Can you work these out from the model? Positions are in its coordinate system, mm. Coordinates: 2 decimals unless noted, no trailing zeros. Order: outer loops, then holes, each group sorted by start corner. A loop starts at its lowest first (then second) coordinate and runs counter-clockwise, first axis right, second up. Notation, with made-up numbers: (43.25, 21.5) -> (101.25, 21.5) arc R10 cw to (101.25, 40.5) -> close; hole circle Ø8 at (-14, 80). An arc over 180 degrees is marked (long way). Return JSON: item names as keys, results as strings. Group by question number.
1) If we section it at B-B, the plane x = 4: Please give me the cut outline in (y, z), then the cut area to 3 significant figures.
2) If we section it at D-D, the plane x = -3.7: Please give me the cut outline in (y, z).
3) If we section it at C-C, the plane z = 1.1: Please give me the cut outline in (x, y).
4) If we section it at A-A, the plane y = -8: Please give me the cut outline in (x, z).
5) If I drill on probe 1 along Y at (x, z) = (-3.7, 1.2); probe 2 along Y at (x, z) = (-3.5, 1.65); probe 3 along X at (y, z) = (13, 0.5), over which ranges is the centre line in solid material (lowest first)? Write a range as from..to.
6) For pin 1 (1 mm diameter, centred on x = -5, z = 2, fed in from +Y); pin 2 (4 mm diameter, centred on x = -3.7, y = 4, fed in from +Z); pin 3 (2.5 mm diameter, centred on x = -3, y = -17, fed in from -Z), each with a flat end and sliding along its axis, tell me the tip position at first contact or that it passes through.
7) Thinking about a two-plate mould opening in X: for faces 1 (the flat face through (0, 0, 2.5)), 2 (the flat face through (4, -17, 1)), 3 (the cylindrical face through (-2.22, 3.39, 1.23)), 4 (the cylindrical face through (-10.14, -24.1, 1.27)), which applies, +X half, -X half, draft (parallel to the pull), parting line (faces both ways), or undercut?
from build123d import *

# Parameters (mm, degrees)
SKETCH_1_W      = 22
SKETCH_1_H      = 50
SKETCH_1_R      = 1.6
EXTRUDE_1_DEPTH = 2.5
CHAMFER_1_SIZE  = 15
FILLET_1_R      = 3


with BuildPart() as part:
    # 草图1 → 凸台-拉伸1 (new body)
    with BuildSketch(Plane.XY):
        Rectangle(SKETCH_1_W, SKETCH_1_H)
        with Locations((-3, -17)):
            Circle(SKETCH_1_R, mode=Mode.SUBTRACT)
        with Locations((3, 17)):
            Circle(SKETCH_1_R, mode=Mode.SUBTRACT)
        with Locations((-3.7, 4)):
            Circle(SKETCH_1_R, mode=Mode.SUBTRACT)
        with Locations((8.3, -8)):
            Circle(SKETCH_1_R, mode=Mode.SUBTRACT)
    extrude(amount=EXTRUDE_1_DEPTH)

    # 倒角1
    chamfer_1_edges = [part.edges().sort_by_distance(p)[0] for p in [
        (11, -25, 1.25),
        (-11, 25, 1.25),
    ]]
    chamfer(chamfer_1_edges, length=CHAMFER_1_SIZE)

    # 圆角1
    fillet_1_edges = [part.edges().sort_by_distance(p)[0] for p in [
        (-11, 10, 1.25),
        (4, 25, 1.25),
        (11, -10, 1.25),
        (-4, -25, 1.25),
        (11, 25, 1.25),
        (-11, -25, 1.25),
    ]]
    fillet(fillet_1_edges, radius=FILLET_1_R)


solid = part.part
Result sheet:
{
 "1": {"outline": "(-17, 0) -> (15.75, 0) -> (15.75, 2.5) -> (-17, 2.5) -> close; (18.25, 0) -> (24.73, 0) -> (24.73, 2.5) -> (18.25, 2.5) -> close", "area": "98.1 mm2"},
 "2": {"outline": "(-24.57, 0) -> (-18.44, 0) -> (-18.44, 2.5) -> (-24.57, 2.5) -> close; (-15.56, 0) -> (2.4, 0) -> (2.4, 2.5) -> (-15.56, 2.5) -> close; (5.6, 0) -> (17.3, 0) -> (17.3, 2.5) -> (5.6, 2.5) -> close"},
 "3": {"outline": "(-11, -22) arc R3 ccw to (-8, -25) -> (-5.24, -25) arc R3 ccw to (-3.12, -24.12) -> (10.12, -10.88) arc R3 ccw to (11, -8.76) -> (11, 22) arc R3 ccw to (8, 25) -> (5.24, 25) arc R3 ccw to (3.12, 24.12) -> (-10.12, 10.88) arc R3 ccw to (-11, 8.76) -> close; hole circle Ø3.2 at (-3.7, 4); hole circle Ø3.2 at (-3, -17); hole circle Ø3.2 at (3, 17); hole circle Ø3.2 at (8.3, -8)"},
 "4": {"outline": "(-11, 0) -> (6.7, 0) -> (6.7, 2.5) -> (-11, 2.5) -> close; (9.9, 0) -> (11, 0) -> (11, 2.5) -> (9.9, 2.5) -> close"},
 "5": {"probe 1": "y = -24.57..-18.44, -15.56..2.4, 5.6..17.3", "probe 2": "y = -24.44..-18.52, -15.48..2.41, 5.59..17.5", "probe 3": "x = -8..11"},
 "6": {"pin 1": "stops at y = 16.5", "pin 2": "stops at z = 2.5", "pin 3": "passes through"},
 "7": {"face 1": "draft", "face 2": "+X half", "face 3": "undercut", "face 4": "-X half"}
}
